```python
from build123d import *

# Parameters (mm, degrees)
BOSS_EXTRUDE1_DEPTH = 1.5


with BuildPart() as part:
    # Sketch1 → Boss-Extrude1 (new, symmetric)
    with BuildSketch(Plane.XY):
        with BuildLine():
            Line((-13.5, 4), (13.5, 4))
            ThreePointArc((13.5, 4), (14.207106781, 4.292893219), (14.5, 5))
            Line((14.5, 5), (14.5, 24))
            Line((14.5, 24), (12, 24))
            Line((12, 24), (14.5, 28))
            Line((14.5, 28), (20.5, 28))
            Line((20.5, 28), (20.5, 2))
            ThreePointArc((20.5, 2), (19.914213562, 0.585786438), (18.5, 0))
            Line((18.5, 0), (-18.5, 0))
            ThreePointArc((-18.5, 0), (-19.914213562, 0.585786438), (-20.5, 2))
            Line((-20.5, 2), (-20.5, 28))
            Line((-20.5, 28), (-14.5, 28))
            Line((-14.5, 28), (-12, 24))
            Line((-12, 24), (-14.5, 24))
            Line((-14.5, 24), (-14.5, 5))
            ThreePointArc((-14.5, 5), (-14.207106781, 4.292893219), (-13.5, 4))
        make_face()
    extrude(amount=BOSS_EXTRUDE1_DEPTH, both=True)


solid = part.part
```
For this review, take the finished solid that the model builds, in its own axes (mm). A direction names the side the tool comes from. Coordinates: 2 decimals unless noted, no trailing zeros. Loops run counter-clockwise (first coordinate to the right, second up) from the corner with the lowest first, then second, coordinate; pieces in that order, holes last.
1. Add section A-A, the plane y = 13.25. Give the boundary of the cut face in (x, z), then the cut area to 3 significant figures.
2. Add section B-B, the plane z = -0.7. Give the boundary of the cut face in (x, y).
3. Add section D-D, the plane y = 26.25. Give the boundary of the cut face in (x, z), then the cut area to 3 significant figures.
4. For line 1 (X direction, y = 16, z = 0.95); line 2 (Y direction, x = 11, z = 1.15); line 3 (X direction, y = 26.25, z = -0.55), list the stretches that pass through material, from the lowest coordinate up.
5. Mouldability with a two-part tool opening along Y and no side actions: class faces 4 (the flat face through (13.23, 25.97, 0.02)), 5 (the flat face through (-14.5, 15, 0)), 6 (the flat face through (20.5, 15, 0)) as +Y half, -Y half, draft (parallel to the pull), parting line (faces both ways), or undercut.
6. Add section C-C, the plane x = 6. Give the boundary of the cut face in (y, z), then the cut area to 3 significant figures.
7. For faces 1 (the flat face through (-13.27, 26.03, 0.02)), 2 (the cylindrical face through (-19.9, 0.57, 0.02)), 3 (the flat face through (13, 24, 0)), list the 3-axis set-ups (+Z, -Z, +X, -X, +Y, -Y) from which the entire face can be reached by the end or side of a thin tool; tool diameter is ignored.
8. Insertion check: P1, Ø1, axis at x = -11.5, y = 22.5, coming from the +Z side; P2, Ø0.9, axis at x = 1.5, z = 0, coming from the +Y side. Each pin has a flat end and moves straight along its axis. Give the tip position at first contact, or say it passes through.
Result:
1. outline: (-20.5, -1.5) - (-14.5, -1.5) - (-14.5, 1.5) - (-20.5, 1.5) - close; (14.5, -1.5) - (20.5, -1.5) - (20.5, 1.5) - (14.5, 1.5) - close
1. area: 36.0 mm2
2. outline: (-20.5, 2) arc R2 ccw to (-18.5, 0) - (18.5, 0) arc R2 ccw to (20.5, 2) - (20.5, 28) - (14.5, 28) - (12, 24) - (14.5, 24) - (14.5, 5) arc R1 cw to (13.5, 4) - (-13.5, 4) arc R1 cw to (-14.5, 5) - (-14.5, 24) - (-12, 24) - (-14.5, 28) - (-20.5, 28) - close
3. outline: (-20.5, -1.5) - (-13.41, -1.5) - (-13.41, 1.5) - (-20.5, 1.5) - close; (13.41, -1.5) - (20.5, -1.5) - (20.5, 1.5) - (13.41, 1.5) - close
3. area: 42.6 mm2
4. line 1: x = -20.5 to -14.5, 14.5 to 20.5
4. line 2: y = 0 to 4
4. line 3: x = -20.5 to -13.41, 13.41 to 20.5
5. face 4: +Y half
5. face 5: undercut
5. face 6: draft
6. outline: (0, -1.5) - (4, -1.5) - (4, 1.5) - (0, 1.5) - close
6. area: 12.0 mm2
7. face 1: +Z, -Z, +Y
7. face 2: +Z, -Z, -X, -Y
7. face 3: +Z, -Z
8. P1: passes through
8. P2: stops at y = 4
